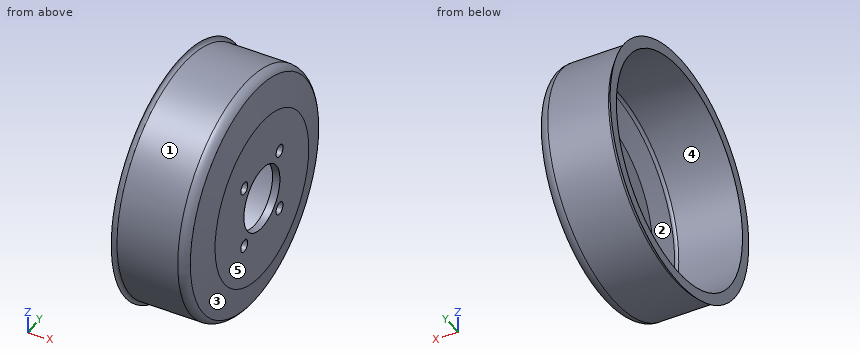
from build123d import *

# Parameters (mm, degrees)
SKETCH2_R          = 5
CUT_EXTRUDE1_DEPTH = 10


with BuildPart() as part:
    # Sketch1 → Revolve1 (revolve)
    with BuildSketch(Plane.XY, mode=Mode.PRIVATE) as revolve1_sk:
        with BuildLine():
            Line((15, 97), (60.316020873, 97))
            Line((60.316020873, 97), (64.382402521, 97))
            ThreePointArc((64.382402521, 97), (68.861218013, 95.806421189), (72.152073668, 92.542269286))
            Line((72.152073668, 92.542269286), (78.152073668, 67.613382081))
            Line((78.152073668, 67.613382081), (78.152073668, 26))
            Line((78.152073668, 26), (72.152073668, 26))
            Line((72.152073668, 26), (72.152073668, 67.613382081))
            Line((72.152073668, 67.613382081), (66.408193592, 89.472988604))
            ThreePointArc((66.408193592, 89.472988604), (65.32157431, 90.589825828), (63.81830321, 91))
            Line((63.81830321, 91), (12, 91))
            Line((12, 91), (12, 100))
            ThreePointArc((12, 100), (12.878679656, 97.878679656), (15, 97))
        make_face()
    revolve(revolve1_sk.sketch.rotate(Axis((-30.728161887, 0, 0), (1, 0, 0)), 90), axis=Axis((-30.728161887, 0, 0), (1, 0, 0)))

    # Sketch2 → Cut-Extrude1 (cut)
    with BuildSketch(Plane(origin=(78.152073668, 0, 0), x_dir=(0, 0, -1), z_dir=(1, 0, 0))):
        with Locations((-25.412524086, 25.499090564)):
            Circle(SKETCH2_R)
        with Locations((25.497475914, 25.414144133)):
            Circle(SKETCH2_R)
        with Locations((25.415769388, -25.495855867)):
            Circle(SKETCH2_R)
        with Locations((-25.494170251, -25.417460204)):
            Circle(SKETCH2_R)
    extrude(amount=-CUT_EXTRUDE1_DEPTH, mode=Mode.SUBTRACT)


solid = part.part
Part model, mm, in its own coordinate system. Face numbers are marked on the shaded views. A direction names the side the tool comes from. Round coordinates to 2 decimals unless told otherwise and drop trailing zeros. Loops run counter-clockwise (first coordinate to the right, second up) from the corner with the lowest first, then second, coordinate; pieces in that order, holes last. Notation, with made-up numbers: (-40, -30) - (-19, -30) arc R20 cw to (-19, -19) - close; hole circle Ø1 at (-4.75, 66.5). An arc over 180 degrees is marked (long way). Answer as a JSON object with one key per item and string values.
Item 1: Wall check: L1, parallel to Y at x = 64, z = -74; L2, parallel to Z at x = 48, y = -10.5; L3, parallel to Z at x = 22.5, y = -51. Give the ranges that are in metal, low to high.
Output:
{"L1": "-62.71 to -52.95, 52.95 to 62.71", "L2": "-96.43 to -90.39, 90.39 to 96.43", "L3": "-82.51 to -75.37, 75.37 to 82.51"}
Item 2: Pin check, flat tips, straight feed: pin 1 (9 mm diameter, centred on y = 25.5, z = 25.41, fed in from +X); pin 2 (13 mm diameter, centred on y = -25.5, z = -25.42, fed in from -X); pin 3 (5 mm diameter, centred on x = 32.5, z = 29, fed in from +Y); pin 4 (4 mm diameter, centred on x = 56.5, y = 24, fed in from +Z). Stop position of each tip, or through.
Output:
{"pin 1": "through", "pin 2": "x = 72.15", "pin 3": "y = 93.31", "pin 4": "z = 94.47"}
Item 3: Tool access for the marked faces 1 and 2: list every direction of +Z, -Z, +X, -X, +Y, -Y with a clear straight run to the whole face (end or side of a thin tool).
Output:
{"face 1": "+X", "face 2": "-X"}
Item 4: Pull direction Z, two halves, no side cores. Call the marked faces 3, 4 and 5: pulls with the +Z half, pulls with the -Z half, needs draft (parallel to the pull), parting line crosses it, or undercut.
Output:
{"face 3": "parting line crosses it", "face 4": "undercut", "face 5": "needs draft"}
Item 5: Band-saw the part on A-A on z = 0. List the corners of the cut face in (x, y).
Output:
{"outline": "(12, -100) arc R3 cw to (15, -97) - (64.38, -97) arc R9 ccw to (72.15, -92.54) - (78.15, -67.61) - (78.15, -26) - (72.15, -26) - (72.15, -67.61) - (66.41, -89.47) arc R2.96 cw to (63.82, -91) - (12, -91) - close; (12, 91) - (63.82, 91) arc R2.96 cw to (66.41, 89.47) - (72.15, 67.61) - (72.15, 26) - (78.15, 26) - (78.15, 67.61) - (72.15, 92.54) arc R9 ccw to (64.38, 97) - (15, 97) arc R3 cw to (12, 100) - close"}
Item 6: Band-saw the part on C-C on x = 41. List the corners of the cut face in (y, z), plus the area to 3 significant figures.
Output:
{"outline": "circle Ø194 at (0, 0); hole circle Ø182 at (0, 0)", "area": "3,540 mm2"}
